```python
from build123d import *

# Parameters (mm, degrees)
F0_W     = 24.2
F0_H     = 16.5
F1_DEPTH = 7
F2_R     = 5.6
F3_W     = 13.1
F3_H     = 13.1
F4_DEPTH = 7.001
F5_W     = 1.05
F5_H     = 13.1
F6_DEPTH = 1.4
F7_R     = 0.6
F8_DEPTH = 7.001
F9_SIZE  = 0.6


with BuildPart() as f1:
    # F0 (on Top) → F1 (new body)
    with BuildSketch(Plane.XY):
        Rectangle(F0_W, F0_H)
    extrude(amount=F1_DEPTH)

    # F2
    f2_edges = [f1.edges().sort_by_distance(p)[0] for p in [
        (-12.1, -8.25, 3.5),
        (12.1, -8.25, 3.5),
        (12.1, 8.25, 3.5),
        (-12.1, 8.25, 3.5),
    ]]
    fillet(f2_edges, radius=F2_R)

    # F3 (on face) → F4 (cut, through all)
    with BuildSketch(Plane(origin=(0, 0, 0), x_dir=(1, 0, 0), z_dir=(0, 0, -1))):
        Rectangle(F3_W, F3_H)
    extrude(amount=-F4_DEPTH, mode=Mode.SUBTRACT)

    # F5 (on face) → F6 (join)
    with BuildSketch(Plane(origin=(0, 0, 0), x_dir=(1, 0, 0), z_dir=(0, 0, -1))):
        with Locations((-6.025, 0)):
            Rectangle(F5_W, F5_H)
        with Locations((6.025, 0)):
            Rectangle(F5_W, F5_H)
    extrude(amount=-F6_DEPTH)

    # F7 (on face) → F8 (cut, through all)
    with BuildSketch(Plane(origin=(0, 0, 0), x_dir=(1, 0, 0), z_dir=(0, 0, -1))):
        with Locations((-9.3, 0)):
            Circle(F7_R)
        with Locations((9.3, 0)):
            Circle(F7_R)
    extrude(amount=-F8_DEPTH, mode=Mode.SUBTRACT)

    # F9
    f9_edges = [f1.edges().sort_by_distance(p)[0] for p in [
        (8.7, 0, 7),
        (-9.9, 0, 7),
    ]]
    chamfer(f9_edges, length=F9_SIZE)


solid = f1.part
```
Geometry check sheet. Reference: the model listing, model coordinates, mm. A direction names the side the tool comes from. Give positions to 0.01 mm unless a question says otherwise; leave off trailing zeros. Order: outer loops, then holes, each group sorted by start corner. A loop starts at its lowest first (then second) coordinate and runs counter-clockwise, first axis right, second up. Notation, with made-up numbers: (59, 62.5) - (72, 62.5) arc R12 ccw to (72, 70.5) - close; hole circle Ø10 at (6.5, 0.25). An arc over 180 degrees is marked (long way). Answer in a Markdown table with one row per item. Add a question column.
Q1. Cross-section at C-C, the plane x = 5.25. Enter the section's corners in (y, z).
Q2. Tool access check on faces 4 (the cylindrical face through (-10.5, -6.57, 3.55)), 5 (the flat face through (-6, 0, 1.4)), 6 (the flat face through (-5.5, 0, 1)). Record the directions out of +Z, -Z, +X, -X, +Y, -Y that give a thin tool (end or side, any length) a straight path to the whole face; none if there is none.
Q3. Cross-section at B-B, the plane y = 0. Enter the section's corners in (x, z), then the cut area to 3 significant figures.
Q4. Gauge pin test, flat ends, axial feed: pin 1 (1 mm diameter, centred on y = 5.5, z = 3, fed in from +X); pin 2 (0.8 mm diameter, centred on x = -6.5, y = 3, fed in from +Z); pin 3 (2 mm diameter, centred on x = 8.5, z = 2, fed in from -Y); pin 4 (0.5 mm diameter, centred on x = 6, y = 0.5, fed in from +Z). Record the tip position at first contact, or that the pin passes through.
Q5. Mould release check, pull along Y, two halves, no side actions. Record for faces 1 (the flat face through (-12.1, 0, 3)), 2 (the cylindrical face through (10.5, 6.57, 3.55)), 3 (the cylindrical face through (-8.746, 0.23, 3.155)): pulls with the +Y half, pulls with the -Y half, needs draft (parallel to the pull), parting line crosses it, or undercut.
Q6. Cross-section at A-A, the plane z = 1. Enter the section's corners in (x, y).
Q7. Material ranges on probe 1 along X at (y, z) = (0, 4); probe 2 along Y at (x, z) = (4.75, 4); probe 3 along X at (y, z) = (-1.75, 5), recorded low to high. Write a range as from..to.
Q8. Cross-section at D-D, the plane y = -4.25. Enter the section's corners in (x, z).
Check values:
| question | item | result |
|---|---|---|
| 1 | outline | (-8.25, 0) - (-6.55, 0) - (-6.55, 7) - (-8.25, 7) - close; (6.55, 0) - (8.25, 0) - (8.25, 7) - (6.55, 7) - close |
| 2 | face 4 | +Z, -Z, -X, -Y |
| 2 | face 5 | +Z |
| 2 | face 6 | +Z, -Z |
| 3 | outline | (-12.1, 0) - (-9.9, 0) - (-9.9, 6.4) - (-10.5, 7) - (-12.1, 7) - close; (-8.7, 0) - (-5.5, 0) - (-5.5, 1.4) - (-6.55, 1.4) - (-6.55, 7) - (-8.1, 7) - (-8.7, 6.4) - close; (5.5, 0) - (8.7, 0) - (8.7, 6.4) - (8.1, 7) - (6.55, 7) - (6.55, 1.4) - (5.5, 1.4) - close; (9.9, 0) - (12.1, 0) - (12.1, 7) - (10.5, 7) - (9.9, 6.4) - close |
| 3 | area | 63.1 mm^2 |
| 4 | pin 1 | stops at x = 11.58 |
| 4 | pin 2 | stops at z = 7 |
| 4 | pin 3 | stops at y = -8.16 |
| 4 | pin 4 | stops at z = 1.4 |
| 5 | face 1 | needs draft |
| 5 | face 2 | pulls with the +Y half |
| 5 | face 3 | undercut |
| 6 | outline | (-12.1, -2.65) arc R5.6 ccw to (-6.5, -8.25) - (6.5, -8.25) arc R5.6 ccw to (12.1, -2.65) - (12.1, 2.65) arc R5.6 ccw to (6.5, 8.25) - (-6.5, 8.25) arc R5.6 ccw to (-12.1, 2.65) - close; hole circle Ø1.2 at (-9.3, 0); hole (-5.5, -6.55) - (5.5, -6.55) - (5.5, 6.55) - (-5.5, 6.55) - close; hole circle Ø1.2 at (9.3, 0) |
| 7 | probe 1 | x = -12.1..-9.9, -8.7..-6.55, 6.55..8.7, 9.9..12.1 |
| 7 | probe 2 | y = -8.25..-6.55, 6.55..8.25 |
| 7 | probe 3 | x = -12.1..-6.55, 6.55..12.1 |
| 8 | outline | (-11.87, 0) - (-5.5, 0) - (-5.5, 1.4) - (-6.55, 1.4) - (-6.55, 7) - (-11.87, 7) - close; (5.5, 0) - (11.87, 0) - (11.87, 7) - (6.55, 7) - (6.55, 1.4) - (5.5, 1.4) - close |
